from build123d import *

# Parameters (mm, degrees)
SKETCH2_W           = 57.8
SKETCH2_H           = 94.8
BOSS_EXTRUDE1_DEPTH = 10
SHELL1_T            = -1
SKETCH3_R           = 8
CUT_EXTRUDE1_DEPTH  = 123.683699502
SKETCH4_R           = 0.5
BOSS_EXTRUDE2_DEPTH = 1


with BuildPart() as part:
    # Sketch2 → Boss-Extrude1 (new body)
    with BuildSketch(Plane(origin=(0, 0, 0), x_dir=(1, 0, 0), z_dir=(0, 1, 0))):
        with Locations((0, 71.411111111)):
            Rectangle(SKETCH2_W, SKETCH2_H)
    extrude(amount=-BOSS_EXTRUDE1_DEPTH)

    # Shell1
    shell1_openings = [part.faces().sort_by_distance(p)[0] for p in [
        (0, -10, -71.411111111),
    ]]
    offset(amount=SHELL1_T, openings=shell1_openings, kind=Kind.INTERSECTION)

    # Sketch3 → Cut-Extrude1 (cut, through all)
    with BuildSketch(Plane(origin=(0, 0, 0), x_dir=(1, 0, 0), z_dir=(0, 1, 0))):
        with Locations(Location((0, 103.340669908, 0), (0, 0, 270))):
            Circle(SKETCH3_R)
    extrude(amount=-CUT_EXTRUDE1_DEPTH, mode=Mode.SUBTRACT)

    # Sketch4 → Boss-Extrude2 (add)
    with BuildSketch(Plane(origin=(28.9, 0, 0), x_dir=(0, 0, -1), z_dir=(1, 0, 0))):
        with Locations((26.011111111, -2)):
            Circle(SKETCH4_R)
    boss_extrude2 = extrude(amount=BOSS_EXTRUDE2_DEPTH)

    # Mirror1: Boss-Extrude2 across plane
    add(boss_extrude2.mirror(Plane(origin=(0, 0, 0), x_dir=(0, 0, 1), z_dir=(1, 0, 0))))


solid = part.part
Design review of the part built by this model. Coordinates are the model's own, in mm. A direction names the side the tool comes from. Round coordinates to 2 decimals unless told otherwise and drop trailing zeros. Loops run counter-clockwise (first coordinate to the right, second up) from the corner with the lowest first, then second, coordinate; pieces in that order, holes last. Notation, with made-up numbers: (26.5, 76) - (85.5, 76) arc R27 cw to (85.5, 98) - close; hole circle Ø5 at (-13, -4.75). An arc over 180 degrees is marked (long way). One line per question, with ' | ' between items.
1. We need section C-C, the plane z = -99. State the section outline as (x, y) points, and give its area (3 significant figures).
Results are:
outline: (-28.9, -10) - (-27.9, -10) - (-27.9, -1) - (-6.72, -1) - (-6.72, 0) - (-28.9, 0) - close; (6.72, -1) - (27.9, -1) - (27.9, -10) - (28.9, -10) - (28.9, 0) - (6.72, 0) - close | area: 62.4 mm²
2. For faces 1 (the face through (-4.87, -0.49, -109.69)), 2 (the face through (27.9, -5, -71)), list the 3-axis set-ups (+Z, -Z, +X, -X, +Y, -Y) from which the entire face can be reached by the end or side of a thin tool; tool diameter is ignored.
Results are:
face 1: +Y, -Y | face 2: -Y
3. For L1, parallel to X at y = -8.25, z = -37; L2, parallel to Z at x = 25, y = -4; L3, parallel to Y at x = 14.5, z = -29, list the stretches that pass through material, from the lowest coordinate up. Write a range as [from, to].
Results are:
L1: x = [-28.9, -27.9], [27.9, 28.9] | L2: z = [-118.81, -117.81], [-25.01, -24.01] | L3: y = [-1, 0]
4. Clearance check with flat-ended pins moving along their axes: P1, Ø2, axis at y = -3, z = -78, coming from the +X side; P2, Ø4, axis at x = -15, z = -81.5, coming from the -Y side; P3, Ø9.5, axis at x = 0, z = -103.34, coming from the +Y side; P4, Ø2.5, axis at y = -5.5, z = -81, coming from the -X side. State where each tip first meets the part, or that it passes through.
Results are:
P1: stops at x = 28.9 | P2: stops at y = -1 | P3: passes through | P4: stops at x = -28.9
5. We need section A-A, the plane x = 0. State the section outline as (y, z) points, and give its area (3 significant figures).
Results are:
outline: (-10, -118.81) - (0, -118.81) - (0, -111.34) - (-1, -111.34) - (-1, -117.81) - (-10, -117.81) - close; (-10, -25.01) - (-1, -25.01) - (-1, -95.34) - (0, -95.34) - (0, -24.01) - (-10, -24.01) - close | area: 96.8 mm²
6. Draft analysis for pull direction Z (two halves, no side actions). For faces 3 (the face through (28.9, -5, -71)), 4 (the face through (-27.9, -5, -71)), 5 (the face through (0, -5, -118.811)), state which applies: released by +Z, released by -Z, zero draft, split by the parting line, or undercut.
Results are:
face 3: zero draft | face 4: undercut | face 5: released by -Z
7. We need section B-B, the plane y = -4.5. State the section outline as (x, z) points.
Results are:
outline: (-28.9, -118.81) - (28.9, -118.81) - (28.9, -24.01) - (-28.9, -24.01) - close; hole (-27.9, -117.81) - (27.9, -117.81) - (27.9, -25.01) - (-27.9, -25.01) - close
8. We need section D-D, the plane x = -16. State the section outline as (y, z) points, and give its area (3 significant figures).
Results are:
outline: (-10, -118.81) - (0, -118.81) - (0, -24.01) - (-10, -24.01) - (-10, -25.01) - (-1, -25.01) - (-1, -117.81) - (-10, -117.81) - close | area: 113 mm²
